Could you check a few things on this model? Use its own coordinates, in mm. Face numbers are marked on the shaded views. A direction names the side the tool comes from. Coordinates: 2 decimals unless noted, no trailing zeros. Order: outer loops, then holes, each group sorted by start corner. A loop starts at its lowest first (then second) coordinate and runs counter-clockwise, first axis right, second up. Notation, with made-up numbers: (8.5, -18.5) - (13.5, -18.5) arc R19 ccw to (13.5, -14.5) - close; hole circle Ø9 at (-26.5, -9.5). An arc over 180 degrees is marked (long way). One line per item, written item: value. Start each with the question number.
from build123d import *

# Parameters (mm, degrees)
SKETCH1_W                                        = 91.44
SKETCH1_H                                        = 38.1
BOSS_EXTRUDE1_DEPTH                              = 3.81
SKETCH2_W                                        = 38.1
SKETCH2_H                                        = 25.4
BOSS_EXTRUDE2_DEPTH                              = 3.81
CBORE_FOR_M3_HEX_HEAD_MACHINE_SCREW1_D           = 3.6
CBORE_FOR_M3_HEX_HEAD_MACHINE_SCREW1_DEPTH       = 3.81
CBORE_FOR_M3_HEX_HEAD_MACHINE_SCREW1_CBORE_D     = 8.4
CBORE_FOR_M3_HEX_HEAD_MACHINE_SCREW1_CBORE_DEPTH = 2.3
FILLET1_R                                        = 6.35
FILLET1_OF_MIRROR1_R                             = 6.35


with BuildPart() as part:
    # Sketch1 → Boss-Extrude1 (new body)
    with BuildSketch(Plane(origin=(0, 0, 0), x_dir=(1, 0, 0), z_dir=(0, 1, 0))):
        Rectangle(SKETCH1_W, SKETCH1_H)
    extrude(amount=BOSS_EXTRUDE1_DEPTH)

    # Sketch2 → Boss-Extrude2 (add)
    with BuildSketch(Plane.ZY.offset(45.72)):
        with Locations((0, 12.7)):
            Rectangle(SKETCH2_W, SKETCH2_H)
    boss_extrude2 = extrude(amount=-BOSS_EXTRUDE2_DEPTH)

    # CBORE for M3 Hex Head Machine Screw1
    with Locations(Plane(origin=(-41.91, 0, 0), x_dir=(0, 0, -1), z_dir=(1, 0, 0))):
        with Locations((-4.939140867, 20.179140867), (4.939140867, 20.179140867), (0, 15.24), (-4.939140867, 10.300859133), (4.939140867, 10.300859133)):
            cbore_for_m3_hex_head_machine_screw1 = CounterBoreHole(CBORE_FOR_M3_HEX_HEAD_MACHINE_SCREW1_D / 2, CBORE_FOR_M3_HEX_HEAD_MACHINE_SCREW1_CBORE_D / 2, CBORE_FOR_M3_HEX_HEAD_MACHINE_SCREW1_CBORE_DEPTH, depth=CBORE_FOR_M3_HEX_HEAD_MACHINE_SCREW1_DEPTH)

    # Fillet1
    fillet1_edges = [part.edges().sort_by_distance(p)[0] for p in [
        (-43.815, 25.4, -19.05),
        (-43.815, 25.4, 19.05),
    ]]
    fillet(fillet1_edges, radius=FILLET1_R)

    # Mirror1: Boss-Extrude2, CBORE for M3 Hex Head Machine Screw1 across plane
    add(boss_extrude2.mirror(Plane(origin=(0, 0, 0), x_dir=(0, 0, 1), z_dir=(1, 0, 0))))
    add(cbore_for_m3_hex_head_machine_screw1.mirror(Plane(origin=(0, 0, 0), x_dir=(0, 0, 1), z_dir=(1, 0, 0))), mode=Mode.SUBTRACT)

    # Fillet1 of Mirror1
    fillet1_of_mirror1_edges = [part.edges().sort_by_distance(p)[0] for p in [
        (43.815, 25.4, -19.05),
        (43.815, 25.4, 19.05),
    ]]
    fillet(fillet1_of_mirror1_edges, radius=FILLET1_OF_MIRROR1_R)


solid = part.part
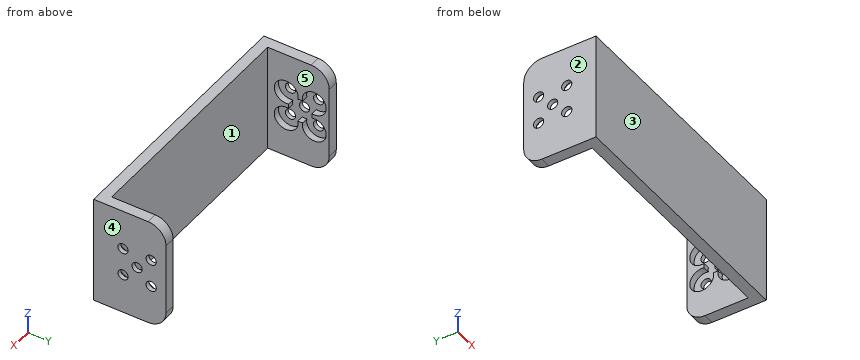
Q1. I want a section at A-A on z = 14.5. Please give me the cut outline in (x, y), then the cut area to 3 significant figures.
Q2. If I drill on L1, parallel to X at y = 4.5, z = 12.5; L2, parallel to X at y = 19.25, z = 7.5; L3, parallel to Y at x = -16.5, z = 13, over which ranges is the centre line in solid material (lowest first)?
Q3. I want a section at B-B on x = -28. Please give me the cut outline in (y, z).
Q4. Which directions (+Z, -Z, +X, -X, +Y, -Y) give clear straight access to the entire face, cutting with the end or side of a thin tool? Please do the marked faces 4 and 5.
Q5. I'm going to push flat-ended pins straight in: pin 1 (3 mm diameter, centred on y = 20.18, z = 4.94, fed in from +X); pin 2 (19 mm diameter, centred on x = -14, z = -2, fed in from +Y). Where does each tip first touch, or does it pass through?
Q6. We'd pull the mould along X, two halves only. Please class the marked faces 1, 2 and 3: +X half, -X half, draft (parallel to the pull), parting line (faces both ways), or undercut.
Values follow:
1. outline: (-45.72, 0) - (45.72, 0) - (45.72, 25.14) - (41.91, 25.14) - (41.91, 3.81) - (-41.91, 3.81) - (-41.91, 25.14) - (-45.72, 25.14) - close
1. area: 511 mm^2
2. L1: x = -45.72 to -41.91, 41.91 to 45.72
2. L2: x = -45.72 to -44.21, 44.21 to 45.72
2. L3: y = 0 to 3.81
3. outline: (0, -19.05) - (3.81, -19.05) - (3.81, 19.05) - (0, 19.05) - close
4. face 4: +Z, -Z, +X, +Y, -Y
4. face 5: +Z, -Z, +Y
5. pin 1: passes through
5. pin 2: stops at y = 3.81
6. face 1: undercut
6. face 2: -X half
6. face 3: draft
